Check sheet for the modelled part. Datum: model origin and axes. Units: mm. Give positions to 0.01 mm unless a question says otherwise; leave off trailing zeros. Order: outer loops, then holes, each group sorted by start corner. A loop starts at its lowest first (then second) coordinate and runs counter-clockwise, first axis right, second up. Notation, with made-up numbers: M 12.25,85 L 22.25,85 A32 ccw 22.25,114 Z; hole C -15.5,53.5 d7. An arc over 180 degrees is marked long. Return JSON: item names as keys, results as strings. Group by question number.
from build123d import *

# Parameters (mm, degrees)
SKETCH_1_W          = 10
SKETCH_1_H          = 1
EXTRUDE_1_DEPTH     = 4
EXTRUDE_2_DEPTH     = 4
EXTRUDE_4_DEPTH     = 4
SKETCH_8_R          = 0.25
CUT_EXTRUDE_1_DEPTH = 10
SKETCH_9_R          = 0.25
CUT_EXTRUDE_2_DEPTH = 10
SCALE_1_SCALE       = 2.454545455


with BuildPart() as part:
    # 草图1 → 凸台-拉伸1 (new body)
    with BuildSketch(Plane(origin=(0, 0, 0), x_dir=(0, 0, -1), z_dir=(1, 0, 0))):
        with Locations((-6.174242424, 5.174378087)):
            Rectangle(SKETCH_1_W, SKETCH_1_H)
    extrude(amount=EXTRUDE_1_DEPTH)

    # 草图4 → 凸台-拉伸2 (add)
    with BuildSketch(Plane(origin=(4, 0, 0), x_dir=(0, 0, -1), z_dir=(1, 0, 0))):
        Polygon((-1.174242424, 5.674378087), (-1.174242424, 4.674378087), (6.675052733, -4.402436637), (6.675052733, -3.402436637), align=None)
    extrude(amount=-EXTRUDE_2_DEPTH)

    # 草图7 → 凸台-拉伸4 (add)
    with BuildSketch(Plane(origin=(4, 0, 0), x_dir=(0, 0, -1), z_dir=(1, 0, 0))):
        with BuildLine():
            Line((-11.174242424, 5.674378087), (-11.174242424, 4.674378087))
            ThreePointArc((-11.174242424, 4.674378087), (-11.674242424, 5.174378087), (-11.174242424, 5.674378087))
        make_face()
    extrude(amount=-EXTRUDE_4_DEPTH)

    # 草图8 → 切除-拉伸1 (cut)
    with BuildSketch(Plane(origin=(4, 0, 0), x_dir=(0, 0, -1), z_dir=(1, 0, 0))):
        with Locations((-11.374242424, 5.174378087)):
            Circle(SKETCH_8_R)
    extrude(amount=-CUT_EXTRUDE_1_DEPTH, mode=Mode.SUBTRACT)

    # 草图9 → 切除-拉伸2 (cut)
    with BuildSketch(Plane(origin=(4, 0, 0), x_dir=(0, 0, -1), z_dir=(1, 0, 0))):
        with Locations((6.403659304, -3.675825169)):
            Circle(SKETCH_9_R)
    extrude(amount=-CUT_EXTRUDE_2_DEPTH, mode=Mode.SUBTRACT)


with BuildPart() as part_1:
    # 缩放比例1: scaled about (2, 3.275952111, 2.445427585)
    add(part.part.scale(SCALE_1_SCALE).moved(Location((-2.909090909, -4.765021252, -3.556985578))))


solid = part_1.part
1) Release check for a two-part mould opening along Z. For faces 1 (the face through (2.069, 7.562, 24.849)), 2 (the face through (2, 6.708, 12)), 3 (the face through (2.07, -14.33, -19.56)), 4 (the face through (2.069, -4.275, -10.173)) record: released by +Z, released by -Z, zero draft, split by the parting line, or undercut.
2) Sectioned sample at C-C on y = -5. Record the boundary of the cut face in (x, z), then the cut area to 3 significant figures.
3) Sectioned sample at B-B on z = 10. Record the boundary of the cut face in (x, y).
4) Sectioned sample at A-A on x = -1.5. Record the boundary of the cut face in (y, z), then the cut area to 3 significant figures.
5) Material ranges on line 1 along Y through (x, z) = (6, 20.5); line 2 along Z through (x, y) = (0.25, 8.25); line 3 along Y through (x, z) = (3, -15.5), recorded low to high.
Reply:
{
 "1": {"face 1": "undercut", "face 2": "zero draft", "face 3": "undercut", "face 4": "released by +Z"},
 "2": {"outline": "M -2.91,-12.92 L 6.91,-12.92 L 6.91,-10.8 L -2.91,-10.8 Z", "area": "20.8 mm^2"},
 "3": {"outline": "M -2.91,6.71 L 6.91,6.71 L 6.91,9.16 L -2.91,9.16 Z"},
 "4": {"outline": "M -15.57,-19.94 L -13.12,-19.94 L 9.16,-0.67 L 9.16,23.87 A1.23 ccw 6.71,23.87 L 6.71,-0.67 Z; hole C -13.79,-19.28 d1.23; hole C 7.94,24.36 d1.23", "area": "108 mm^2"},
 "5": {"line 1": "6.71 to 9.16", "line 2": "-1.46 to 23.83, 24.89 to 25.06", "line 3": "-10.44 to -7.98"}
}
